Work out the finished part from the listing and answer in its coordinate system (mm). Face numbers are marked on the shaded views. A direction names the side the tool comes from. Coordinates: 2 decimals unless noted, no trailing zeros. Write each loop counter-clockwise with the first axis right and the second up, starting at its lowest first coordinate (ties: lowest second). Pieces come first, ordered by that corner, then holes. Notation, with made-up numbers: (7.25, -2) - (15.25, -2) arc R24 ccw to (15.25, 17) - close; hole circle Ø11 at (-39.5, -23.5). An arc over 180 degrees is marked (long way). Answer as a JSON object with one key per item and string values. Group by question number.
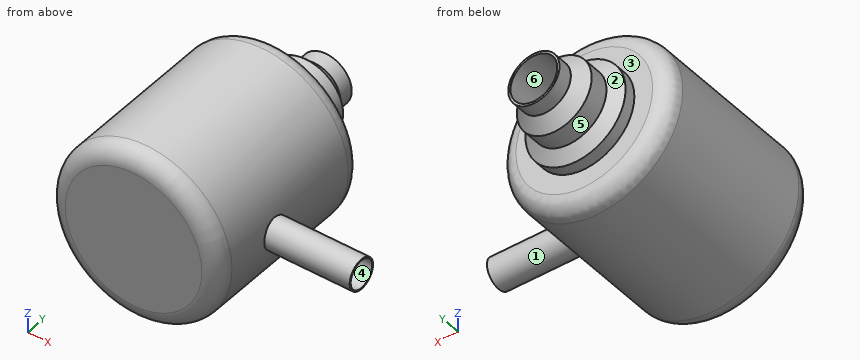
from build123d import *

# Parameters (mm, degrees)
SKETCH2_R           = 2.5
BOSS_EXTRUDE1_DEPTH = 5
SKETCH4_R           = 0.684081367
CUT_EXTRUDE1_DEPTH  = 5
FILLET2_R           = 0.5
SKETCH5_R           = 0.45
BOSS_EXTRUDE2_DEPTH = 5
SKETCH6_R           = 0.411041126
CUT_EXTRUDE2_DEPTH  = 4


with BuildPart() as part:
    # Sketch2 → Boss-Extrude1 (new body)
    with BuildSketch(Plane(origin=(0, 0, 0), x_dir=(1, 0, 0), z_dir=(0, 1, 0))):
        Circle(SKETCH2_R)
    extrude(amount=BOSS_EXTRUDE1_DEPTH)

    # Sketch3 → Revolve2 (revolve)
    with BuildSketch(Plane.XY):
        Polygon((0, 7.411705002), (-0.75, 7.411705002), (-0.75, 6.975061564), (-1.095892568, 6.629168996), (-1.095892568, 6.058427362), (-1.465907088, 5.809167185), (-1.465907088, 5.471459847), (-2.5, 5.471459847), (-2.5, 5), (0, 5), align=None)
    revolve(axis=Axis((0, 0, 0), (0, 1, 0)))

    # Sketch4 → Cut-Extrude1 (cut)
    with BuildSketch(Plane(origin=(0, 7.411705002, 0), x_dir=(1, 0, 0), z_dir=(0, 1, 0))):
        Circle(SKETCH4_R)
    extrude(amount=-CUT_EXTRUDE1_DEPTH, mode=Mode.SUBTRACT)

    # Fillet2
    fillet2_edges = [part.edges().sort_by_distance(p)[0] for p in [
        (-2.5, 0, 0),
        (2.5, 5.471459847, 0),
    ]]
    fillet(fillet2_edges, radius=FILLET2_R)

    # Sketch5 → Boss-Extrude2 (add)
    with BuildSketch(Plane(origin=(0, 0, 0), x_dir=(0, 0, -1), z_dir=(1, 0, 0))):
        with Locations((0, 2.194655863)):
            Circle(SKETCH5_R)
    extrude(amount=BOSS_EXTRUDE2_DEPTH)

    # Sketch6 → Cut-Extrude2 (cut)
    with BuildSketch(Plane(origin=(5, 0, 0), x_dir=(0, 0, -1), z_dir=(1, 0, 0))):
        with Locations((0, 2.194655863)):
            Circle(SKETCH6_R)
    extrude(amount=-CUT_EXTRUDE2_DEPTH, mode=Mode.SUBTRACT)


solid = part.part
Q1. A tool of negligible diameter and unlimited length cuts with its end or side. For the marked faces 1 and 2, from which of +Z, -Z, +X, -X, +Y, -Y can it reach the whole face along a straight path? Write none if from no direction.
Q2. For a pull along Z with two mould halves and no side action, classify the marked faces 3, 4, 5 and 6 as +Z half, -Z half, draft (parallel to the pull), parting line (faces both ways), or undercut.
Q3. Flat-ended cylindrical pins translate along their axes: pin 1 Ø3 at (y, z) = (3.5, 2) entering from +X; pin 2 Ø2 at (x, y) = (3.5, 6.5) entering from +Z; pin 3 Ø2 at (y, z) = (5, 1) entering from +X. Find the tip coordinate at first contact, or state that the pin passes through.
Q4. Consider L1, parallel to Z at x = 0, y = 6.3; L2, parallel to Z at x = 1.5, y = 1; L3, parallel to Y at x = 1.5, z = -0.2. Determine where each line is inside the solid, lowest interval first. Write a range as from..to.
Q5. Section A-A on y = 1 is taken. Determine the outline of the cut face in (x, z), plus the area to 3 significant figures.
Q6. Section B-B on x = 4.25 is taken. Determine the outline of the cut face in (y, z).
Numbers:
{
 "1": {"face 1": "+X", "face 2": "+Y"},
 "2": {"face 3": "draft", "face 4": "undercut", "face 5": "parting line", "face 6": "undercut"},
 "3": {"pin 1": "stops at x = 2.45", "pin 2": "passes through", "pin 3": "stops at x = 2.5"},
 "4": {"L1": "z = -1.1..-0.68, 0.68..1.1", "L2": "z = -2..2", "L3": "y = 0..1.84, 2.55..5.47"},
 "5": {"outline": "circle Ø5 at (0, 0)", "area": "19.6 mm²"},
 "6": {"outline": "circle Ø0.9 at (2.19, 0); hole circle Ø0.82 at (2.19, 0)"}
}
